Read the model definition and answer for the solid it produces. Units are mm, in the model's axes. Face numbers are marked on the shaded views. A direction names the side the tool comes from. Give positions to 0.01 mm unless a question says otherwise; leave off trailing zeros. Order: outer loops, then holes, each group sorted by start corner. A loop starts at its lowest first (then second) coordinate and runs counter-clockwise, first axis right, second up. Notation, with made-up numbers: (73.25, -18.5) - (82.25, -18.5) arc R13 cw to (82.25, 6.5) - close; hole circle Ø7 at (-10, -29.75). An arc over 180 degrees is marked (long way). Write each question's results on one line, items separated by ' | '. Start each with the question number.
Q1. Flat-ended cylindrical pins translate along their axes: P1, Ø1.8, axis at y = 74.5, z = 4, coming from the +X side; P2, Ø2.5, axis at x = 0, y = 0, coming from the -Z side; P3, Ø2, axis at x = -8.5, z = 1.5, coming from the -Y side; P4, Ø1.2, axis at y = 73, z = 3.5, coming from the -X side. Find the tip coordinate at first contact, or state that the pin passes through.
Q2. A tool of negligible diameter and unlimited length cuts with its end or side. For the marked faces 1, 2 and 3, from which of +Z, -Z, +X, -X, +Y, -Y can it reach the whole face along a straight path? Write none if from no direction.
Q3. Find the intervals of material crossed by line 1 along Z through (x, y) = (0, 68.8); line 2 along Y through (x, z) = (-0.5, 0.5); line 3 along Y through (x, z) = (0, 2.7), in increasing order. Write a range as from..to.
Q4. Find section B-B on x = 0. Give the vertices of the cut face in (y, z).
Q5. Find section C-C on y = 53.5. Give the vertices of the cut face in (x, z).
Q6. Find section A-A on z = 3. Give the vertices of the cut face in (x, y), and give its area (3 significant figures).
Q7. Find section D-D on x = -4.5. Give the vertices of the cut face in (y, z), and give its area (3 significant figures).
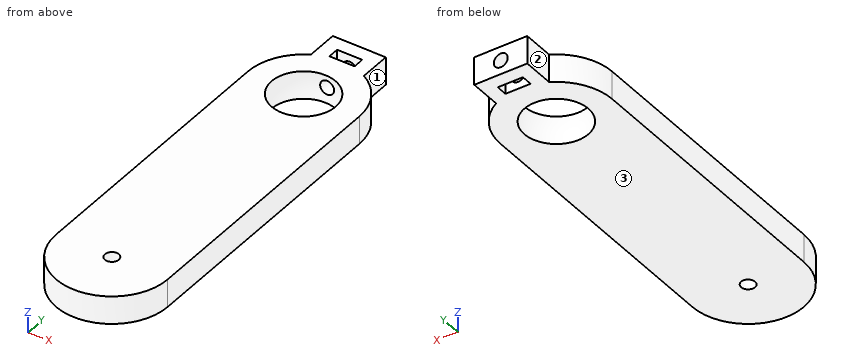
from build123d import *

# Parameters (mm, degrees)
F0_R     = 1.5
F1_DEPTH = 6
F3_W     = 11.4
F3_H     = 9.9
F3_W_2   = 5.4
F3_H_2   = 2.4
F4_DEPTH = 6
F6_R     = 1.5
F7_DEPTH = 11.0515308717


with BuildPart() as f1:
    # F0 (on Top) → F1 (new body)
    with BuildSketch(Plane.XY):
        with BuildLine():
            Line((-12, 60), (-12, 0))
            ThreePointArc((-12, 0), (0, -12), (12, 0))
            Line((12, 0), (12, 60))
            ThreePointArc((12, 60), (0, 72), (-12, 60))
        make_face()
        Circle(F0_R, mode=Mode.SUBTRACT)
    extrude(amount=F1_DEPTH)

    # F3 (on face) → F4 (join, through all)
    with BuildSketch(Plane(origin=(0, 0, 0), x_dir=(1, 0, 0), z_dir=(0, 0, -1))):
        with Locations((0, -72.45)):
            Rectangle(F3_W, F3_H)
        with Locations((0, -73.2)):
            Rectangle(F3_W_2, F3_H_2, mode=Mode.SUBTRACT)
    extrude(amount=-F4_DEPTH)

    # F2 (on Right) → F5 (revolve, cut)
    with BuildSketch(Plane.YZ):
        with BuildLine():
            ThreePointArc((60, -4.5), (67.5, 3), (60, 10.5))
            Line((60, 10.5), (60, -4.5))
        make_face()
    revolve(axis=Axis((0, 60, 3), (0, 0, -1)), mode=Mode.SUBTRACT)

    # F6 (on face) → F7 (cut, up to face)
    with BuildSketch(Plane(origin=(0, 77.4, 0), x_dir=(-1, 0, 0), z_dir=(0, 1, 0))):
        with Locations((0, 3)):
            Circle(F6_R)
    extrude(amount=-F7_DEPTH, mode=Mode.SUBTRACT)


solid = f1.part
Working result:
1) P1: x = 5.7 | P2: through | P3: y = -9.37 | P4: x = -5.7
2) face 1: +Z, -Z, +X, +Y | face 2: +Z, -Z, -X, +Y | face 3: -Z, +X, -X, +Y, -Y
3) line 1: 0..1.5, 4.5..6 | line 2: -11.99..-1.41, 1.41..52.95, 67.05..72, 74.4..77.4 | line 3: -12..-1.5, 1.5..52.51
4) outline: (-12, 0) - (-1.5, 0) - (-1.5, 6) - (-12, 6) - close; (1.5, 0) - (53.13, 0) arc R7.5 cw to (53.13, 6) - (1.5, 6) - close; (66.87, 0) - (72, 0) - (72, 1.5) - (67.35, 1.5) arc R7.5 cw to start; (66.87, 6) arc R7.5 cw to (67.35, 4.5) - (72, 4.5) - (72, 6) - close; (74.4, 0) - (77.4, 0) - (77.4, 1.5) - (74.4, 1.5) - close; (74.4, 4.5) - (77.4, 4.5) - (77.4, 6) - (74.4, 6) - close
5) outline: (-12, 0) - (-2.24, 0) arc R3.74 cw to (-2.24, 6) - (-12, 6) - close; (2.24, 0) - (12, 0) - (12, 6) - (2.24, 6) arc R3.74 cw to start
6) outline: (-12, 0) arc R12 ccw to (12, 0) - (12, 60) arc R12 ccw to (5.7, 70.56) - (5.7, 77.4) - (1.5, 77.4) - (1.5, 74.4) - (2.7, 74.4) - (2.7, 72) - (1.5, 72) - (1.5, 67.35) arc R7.5 cw (long way) to (-1.5, 67.35) - (-1.5, 72) - (-2.7, 72) - (-2.7, 74.4) - (-1.5, 74.4) - (-1.5, 77.4) - (-5.7, 77.4) - (-5.7, 70.56) arc R12 ccw to (-12, 60) - close; hole circle Ø3 at (0, 0) | area: 1,740 mm²
7) outline: (-11.12, 0) - (54.8, 0) arc R6 cw to (54.8, 6) - (-11.12, 6) - close; (65.2, 0) - (77.4, 0) - (77.4, 6) - (65.2, 6) arc R6 cw to start | area: 462 mm²
